from build123d import *

# Parameters (mm, degrees)
SKETCH_1_R          = 13.5
EXTRUDE_1_DEPTH     = 6
SKETCH_3_R          = 1.5
CUT_EXTRUDE_2_DEPTH = 21.012496096
CUT_EXTRUDE_START   = -3
SKETCH_4_R          = 13.5
SKETCH_4_R_2        = 9
CUT_EXTRUDE_3_DEPTH = 3


with BuildPart() as part:
    # 草图1 → 凸台-拉伸1 (new body)
    with BuildSketch(Plane.XY):
        Circle(SKETCH_1_R)
    extrude(amount=EXTRUDE_1_DEPTH)

    # 草图3 → 切除-拉伸2 (cut, through all)
    with BuildSketch(Plane.XY):
        Circle(SKETCH_3_R)
    extrude(amount=CUT_EXTRUDE_2_DEPTH, mode=Mode.SUBTRACT)

    # 草图4 → 切除-拉伸3 (cut)
    with BuildSketch(Plane.XY.offset(4.5).offset(CUT_EXTRUDE_START)):
        Circle(SKETCH_4_R)
        Circle(SKETCH_4_R_2, mode=Mode.SUBTRACT)
    extrude(amount=CUT_EXTRUDE_3_DEPTH, mode=Mode.SUBTRACT)


solid = part.part
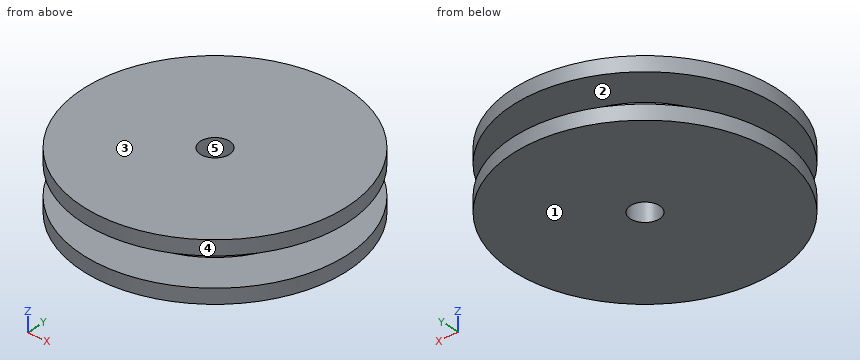
Part model, mm, in its own coordinate system. Face numbers are marked on the shaded views. A direction names the side the tool comes from. Coordinates: 2 decimals unless noted, no trailing zeros. Write each loop counter-clockwise with the first axis right and the second up, starting at its lowest first coordinate (ties: lowest second). Pieces come first, ordered by that corner, then holes. Notation, with made-up numbers: (-28, -22.5) - (-18, -22.5) arc R18 ccw to (-18, -11.5) - close; hole circle Ø3 at (76, 20.5). An arc over 180 degrees is marked (long way). Put each result on its own line as item: value.
1. Band-saw the part on D-D (x = -10.25). Write the cut outline in (y, z).
Final values:
outline: (-8.79, 0) - (8.79, 0) - (8.79, 1.5) - (-8.79, 1.5) - close; (-8.79, 4.5) - (8.79, 4.5) - (8.79, 6) - (-8.79, 6) - close
2. Band-saw the part on C-C (z = 2.9). Write the cut outline in (x, y).
Final values:
outline: circle Ø18 at (0, 0); hole circle Ø3 at (0, 0)
3. Probe line 1 along Z through (x, y) = (-9.5, -3); line 2 along Y through (x, z) = (0, 2.8); line 3 along Y through (x, z) = (0.5, 5.55). List the from-to ranges inside material, lowest first. Write a range as [from, to].
Final values:
line 1: z = [0, 1.5], [4.5, 6]
line 2: y = [-9, -1.5], [1.5, 9]
line 3: y = [-13.49, -1.41], [1.41, 13.49]
4. 3-axis set-ups, long thin cutter, end or side, ignore diameter. For the marked faces 1 and 2: which of +Z, -Z, +X, -X, +Y, -Y reach the whole face in a straight line?
Final values:
face 1: -Z, +X, -X, +Y, -Y
face 2: none
5. Flat gauge pin, fed straight in: pin 1 Ø3 at (y, z) = (-7.5, 4.5) entering from +X. Where does the tip first touch, or does it go through?
Final values:
pin 1: stops at x = 12.09
6. Band-saw the part on A-A (y = 0). Write the cut outline in (x, z).
Final values:
outline: (-13.5, 0) - (-1.5, 0) - (-1.5, 6) - (-13.5, 6) - (-13.5, 4.5) - (-9, 4.5) - (-9, 1.5) - (-13.5, 1.5) - close; (1.5, 0) - (13.5, 0) - (13.5, 1.5) - (9, 1.5) - (9, 4.5) - (13.5, 4.5) - (13.5, 6) - (1.5, 6) - close
7. Two-plate mould, pull along X, no slides. Class the marked faces 3, 4 and 5: +X half, -X half, draft (parallel to the pull), parting line (faces both ways), or undercut.
Final values:
face 3: draft
face 4: parting line
face 5: undercut
